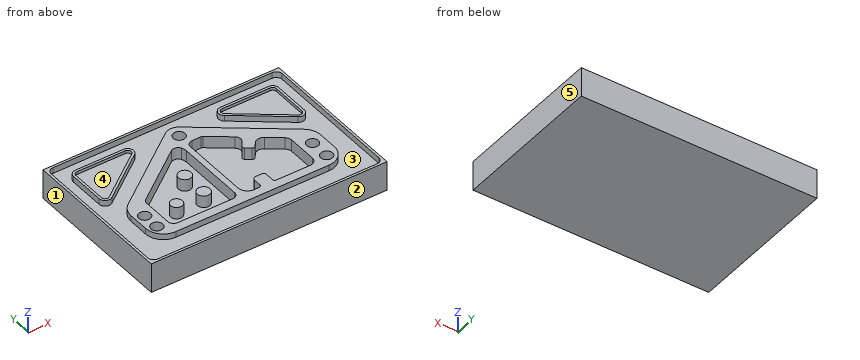
```python
from build123d import *

# Parameters (mm, degrees)
BASE_TRIANGLE_DEPTH  = 50
SKETCH5_W            = 400
SKETCH5_H            = 260
BASE_RECTANGLE_DEPTH = 40
POCKETS_DEPTH        = 20
SKETCH3_R            = 10
CUT_HOLES_DEPTH      = 40
SKETCH4_R            = 10.786602673
SKETCH4_R_2          = 10
POCKET_BOSS_DEPTH    = 20
SKETCH6_W            = 400
SKETCH6_H            = 260
RIM_DEPTH            = 10
TRI_BOSS_DEPTH       = 10
TRI_POCK_S_DEPTH     = 5


with BuildPart() as part:
    # Sketch1 → Base - Triangle (new body)
    with BuildSketch(Plane.XY):
        with BuildLine():
            Line((-13.666666667, 109.75), (-148, 9))
            ThreePointArc((-148, 9), (-156.83281573, -1.583592135), (-160, -15))
            Line((-160, -15), (-160, -50))
            ThreePointArc((-160, -50), (-151.213203436, -71.213203436), (-130, -80))
            Line((-130, -80), (130, -80))
            ThreePointArc((130, -80), (151.213203436, -71.213203436), (160, -50))
            Line((160, -50), (160, -17.5))
            ThreePointArc((160, -17.5), (156.83281573, -4.083592135), (148, 6.5))
            Line((148, 6.5), (10.333333333, 109.75))
            ThreePointArc((10.333333333, 109.75), (-1.666666667, 113.75), (-13.666666667, 109.75))
        make_face()
    extrude(amount=BASE_TRIANGLE_DEPTH)

    # Sketch5 → Base - Rectangle (add)
    with BuildSketch(Plane.XY):
        with Locations((0, 10)):
            Rectangle(SKETCH5_W, SKETCH5_H)
    extrude(amount=BASE_RECTANGLE_DEPTH)

    # Sketch2 → Pockets (cut)
    with BuildSketch(Plane.XY.offset(50)):
        with BuildLine():
            Line((-126.20392244, -4.65294183), (-126.20392244, -55.061436747))
            ThreePointArc((-126.20392244, -55.061436747), (-123.274990252, -62.132504559), (-116.20392244, -65.061436747))
            Line((-116.20392244, -65.061436747), (-22.729187789, -65.061436747))
            ThreePointArc((-22.729187789, -65.061436747), (-15.658119977, -62.132504559), (-12.729187789, -55.061436747))
            Line((-12.729187789, -55.061436747), (-12.729187789, 60.20056332))
            ThreePointArc((-12.729187789, 60.20056332), (-13.262082788, 64.786609863), (-14.832370079, 69.12826828))
            ThreePointArc((-14.832370079, 69.12826828), (-21.478744287, 74.395841003), (-29.780778934, 72.6644158))
            Line((-29.780778934, 72.6644158), (-122.20392244, 3.34705817))
            ThreePointArc((-122.20392244, 3.34705817), (-125.14819435, -0.180805875), (-126.20392244, -4.65294183))
        make_face()
        with BuildLine():
            Line((-2.969097688, 64.72393548), (-2.969097688, -49.319676422))
            ThreePointArc((-2.969097688, -49.319676422), (1.717193813, -60.633384921), (13.030902312, -65.319676422))
            Line((13.030902312, -65.319676422), (22.011923396, -65.319676422))
            ThreePointArc((22.011923396, -65.319676422), (24.840350521, -64.148103547), (26.011923396, -61.319676422))
            Line((26.011923396, -61.319676422), (26.011923396, -48.319676422))
            ThreePointArc((26.011923396, -48.319676422), (27.769282709, -44.077035735), (32.011923396, -42.319676422))
            Line((32.011923396, -42.319676422), (43.011923396, -42.319676422))
            ThreePointArc((43.011923396, -42.319676422), (45.840350521, -43.491249298), (47.011923396, -46.319676422))
            Line((47.011923396, -46.319676422), (47.011923396, -61.319676422))
            ThreePointArc((47.011923396, -61.319676422), (48.183496271, -64.148103547), (51.011923396, -65.319676422))
            Line((51.011923396, -65.319676422), (108.417947751, -65.319676422))
            ThreePointArc((108.417947751, -65.319676422), (116.903229125, -61.804957797), (120.417947751, -53.319676422))
            Line((120.417947751, -53.319676422), (120.417947751, -3.813460813))
            ThreePointArc((120.417947751, -3.813460813), (119.151074043, 1.553102333), (115.617947751, 5.786539187))
            Line((115.617947751, 5.786539187), (92.782280857, 22.913289357))
            ThreePointArc((92.782280857, 22.913289357), (84.071541357, 25.217812286), (76.212563172, 20.810514877))
            Line((76.212563172, 20.810514877), (70.571566089, 13.760633559))
            ThreePointArc((70.571566089, 13.760633559), (67.951906694, 12.291534423), (65.04832686, 13.059708732))
            Line((65.04832686, 13.059708732), (56.830014172, 19.223443248))
            ThreePointArc((56.830014172, 19.223443248), (55.270216198, 21.857757823), (56.030014172, 24.823443248))
            Line((56.030014172, 24.823443248), (62.343956311, 33.242032767))
            ThreePointArc((62.343956311, 33.242032767), (64.243451248, 40.656246329), (60.343956311, 47.242032767))
            Line((60.343956311, 47.242032767), (24.768086026, 73.92393548))
            ThreePointArc((24.768086026, 73.92393548), (23.63299709, 74.518668672), (22.368086026, 74.72393548))
            Line((22.368086026, 74.72393548), (7.030902312, 74.72393548))
            ThreePointArc((7.030902312, 74.72393548), (-0.0401655, 71.795003292), (-2.969097688, 64.72393548))
        make_face()
    extrude(amount=-POCKETS_DEPTH, mode=Mode.SUBTRACT)

    # Sketch3 → Cut - Holes (cut)
    with BuildSketch(Plane.XY.offset(50)):
        with Locations((-144.880429534, -26.083370712)):
            Circle(SKETCH3_R)
        with Locations((-144.880429534, -55.454261033)):
            Circle(SKETCH3_R)
        with Locations((140, -26.083370712)):
            Circle(SKETCH3_R)
        with Locations((140, -60)):
            Circle(SKETCH3_R)
        with Locations((-1.666666667, 93.75)):
            Circle(SKETCH3_R)
    extrude(amount=-CUT_HOLES_DEPTH, mode=Mode.SUBTRACT)

    # Sketch4 → Pocket Boss (add)
    with BuildSketch(Plane.XY.offset(30)):
        with Locations(Location((-46.246176072, 17.161613861, 0), (0, 0, 180))):
            Circle(SKETCH4_R)
        with Locations(Location((-46.246176072, -28.171767173, 0), (0, 0, 180))):
            Circle(SKETCH4_R)
        with Locations(Location((-92.222494778, -28.171767173, 0), (0, 0, 180))):
            Circle(SKETCH4_R_2)
    extrude(amount=POCKET_BOSS_DEPTH)

    # Sketch6 → Rim (add)
    with BuildSketch(Plane.XY.offset(40)):
        with Locations((0, 10)):
            Rectangle(SKETCH6_W, SKETCH6_H)
        with BuildLine():
            Line((-196, 126), (-196, -106))
            ThreePointArc((-196, -106), (-193.071067812, -113.071067812), (-186, -116))
            Line((-186, -116), (186, -116))
            ThreePointArc((186, -116), (193.071067812, -113.071067812), (196, -106))
            Line((196, -106), (196, 126))
            ThreePointArc((196, 126), (193.071067812, 133.071067812), (186, 136))
            Line((186, 136), (-186, 136))
            ThreePointArc((-186, 136), (-193.071067812, 133.071067812), (-196, 126))
        make_face(mode=Mode.SUBTRACT)
    extrude(amount=RIM_DEPTH)

    # Sketch7 → Tri - Boss (add)
    with BuildSketch(Plane.XY.offset(40)):
        with BuildLine():
            Line((-164, 113.448068866), (-82.069241512, 113.448068866))
            ThreePointArc((-82.069241512, 113.448068866), (-72.582408532, 106.610346526), (-76.069241512, 95.448068866))
            Line((-76.069241512, 95.448068866), (-158, 34))
            ThreePointArc((-158, 34), (-168.472135955, 33.05572809), (-174, 42))
            Line((-174, 42), (-174, 103.448068866))
            ThreePointArc((-174, 103.448068866), (-171.071067812, 110.519136678), (-164, 113.448068866))
        make_face()
        with BuildLine():
            Line((158, 34), (76.069241512, 95.448068866))
            ThreePointArc((76.069241512, 95.448068866), (72.582408532, 106.610346526), (82.069241512, 113.448068866))
            Line((82.069241512, 113.448068866), (164, 113.448068866))
            ThreePointArc((164, 113.448068866), (171.071067812, 110.519136678), (174, 103.448068866))
            Line((174, 103.448068866), (174, 42))
            ThreePointArc((174, 42), (168.472135955, 33.05572809), (158, 34))
        make_face()
    extrude(amount=TRI_BOSS_DEPTH)

    # Sketch8 → Tri - Pock_s (cut)
    with BuildSketch(Plane.XY.offset(50)):
        with BuildLine():
            Line((-82.069241512, 109.448068866), (-164, 109.448068866))
            ThreePointArc((-164, 109.448068866), (-168.242640687, 107.690709553), (-170, 103.448068866))
            Line((-170, 103.448068866), (-170, 42))
            ThreePointArc((-170, 42), (-166.683281573, 36.633436854), (-160.4, 37.2))
            Line((-160.4, 37.2), (-78.469241512, 98.648068866))
            ThreePointArc((-78.469241512, 98.648068866), (-76.377141724, 105.345435462), (-82.069241512, 109.448068866))
        make_face()
        with BuildLine():
            Line((170, 42), (170, 103.448068866))
            ThreePointArc((170, 103.448068866), (168.242640687, 107.690709553), (164, 109.448068866))
            Line((164, 109.448068866), (82.069241512, 109.448068866))
            ThreePointArc((82.069241512, 109.448068866), (76.377141724, 105.345435462), (78.469241512, 98.648068866))
            Line((78.469241512, 98.648068866), (160.4, 37.2))
            ThreePointArc((160.4, 37.2), (166.683281573, 36.633436854), (170, 42))
        make_face()
    extrude(amount=-TRI_POCK_S_DEPTH, mode=Mode.SUBTRACT)


solid = part.part
```
The listing builds one solid part. Answer for the finished solid, in the listing's coordinates (mm). Face numbers are marked on the shaded views. A direction names the side the tool comes from. Give positions to 0.01 mm unless a question says otherwise; leave off trailing zeros. Loops run counter-clockwise (first coordinate to the right, second up) from the corner with the lowest first, then second, coordinate; pieces in that order, holes last. Notation, with made-up numbers: (41.25, 39.5) - (87.25, 39.5) arc R18 ccw to (87.25, 60.5) - close; hole circle Ø11 at (-4, -38). An arc over 180 degrees is marked (long way). Answer as CSV lines item,"result". Start each with the question number.
Item 1: The mould has two halves that part along Y. Classify the marked faces 1, 2 and 3: +Y half, -Y half, draft (parallel to the pull), parting line (faces both ways), or undercut.
Item 2: For the marked faces 4 and 5, determine the directions among +Z, -Z, +X, -X, +Y, -Y from which every point of the face is accessible in a straight line to the end or side of a thin tool.
Item 3: A cutting plane is placed at A-A on y = -89. Determine the outline of the cut face in (x, z).
Item 4: A cutting plane is placed at C-C on y = -8.5. Determine the outline of the cut face in (x, z), then the cut area to 3 significant figures.
Item 5: A cutting plane is placed at B-B on x = 140. Determine the outline of the cut face in (y, z).
Item 6: Find the intervals of material crossed by line 1 (Y direction, x = 140, z = 28); line 2 (X direction, y = 27, z = 30.5); line 3 (Y direction, x = 122, z = 42), in increasing order. Write a range as from..to.
Item 7: Each of these flat-tipped pins is pushed along its axis until it touches: pin 1 (23 mm diameter, centred on x = -1.67, y = 93.75, fed in from +Z); pin 2 (6 mm diameter, centred on x = -37, y = -38.5, fed in from +Z). Where does it stop, or does it pass through?
Found:
1,face 1,"draft"
1,face 2,"-Y half"
1,face 3,"undercut"
2,face 4,"+Z"
2,face 5,"+Z, -Z, +X, +Y, -Y"
3,outline,"(-200, 0) - (200, 0) - (200, 50) - (196, 50) - (196, 40) - (-196, 40) - (-196, 50) - (-200, 50) - close"
4,outline,"(-200, 0) - (200, 0) - (200, 50) - (196, 50) - (196, 40) - (158.62, 40) - (158.62, 50) - (120.42, 50) - (120.42, 30) - (-2.97, 30) - (-2.97, 50) - (-12.73, 50) - (-12.73, 30) - (-126.2, 30) - (-126.2, 50) - (-159.29, 50) - (-159.29, 40) - (-196, 40) - (-196, 50) - (-200, 50) - close"
4,area,"14,500 mm^2"
5,outline,"(-120, 0) - (140, 0) - (140, 50) - (136, 50) - (136, 40) - (113.45, 40) - (113.45, 50) - (109.45, 50) - (109.45, 45) - (52.5, 45) - (52.5, 50) - (47.5, 50) - (47.5, 40) - (12.5, 40) - (12.5, 50) - (-16.08, 50) - (-16.08, 10) - (-36.08, 10) - (-36.08, 50) - (-50, 50) - (-50, 10) - (-70, 10) - (-70, 50) - (-78.28, 50) - (-78.28, 40) - (-116, 40) - (-116, 50) - (-120, 50) - close"
6,line 1,"y = -120..-70, -50..-36.08, -16.08..140"
6,line 2,"x = -200..-90.67, -50.67..-41.82, -12.73..-2.97, 57.66..200"
6,line 3,"y = -120..-116, -80..26, 61..113.45, 136..140"
7,pin 1,"stops at z = 50"
7,pin 2,"stops at z = 30"
